```python
from build123d import *

# Parameters (mm, degrees)
SCHIZZO1_R          = 7
ESTRUSIONE1_DEPTH   = 20
SCHIZZO2_R          = 6
ESTRUSIONE2_DEPTH   = 12
ESTRUSIONE3_DEPTH   = 8
SCHIZZO4_OUTSIDE_W  = 31.456
SCHIZZO4_OUTSIDE_H  = 33.832
SCHIZZO4_OUTSIDE_R  = 5.5
ESTRUSIONE4_DEPTH   = 4
SMUSSO1_SIZE        = 0.5
SMUSSO1_EDGE_2_SIZE = 0.5
SMUSSO1_EDGE_3_SIZE = 0.5
SMUSSO1_EDGE_4_SIZE = 0.5
SMUSSO1_EDGE_5_SIZE = 0.5
SMUSSO1_EDGE_6_SIZE = 0.5
SMUSSO2_SIZE        = 1
RACCORDO1_R         = 2
RACCORDO2_R         = 0.5
SMUSSO3_SIZE        = 1


with BuildPart() as part:
    # Schizzo1 → Estrusione1 (new body)
    with BuildSketch(Plane(origin=(0, 0, 0), x_dir=(0, 0, -1), z_dir=(1, 0, 0))):
        Circle(SCHIZZO1_R)
    extrude(amount=ESTRUSIONE1_DEPTH)

    # Schizzo2 → Estrusione2 (add)
    with BuildSketch(Plane(origin=(20, 0, 0), x_dir=(0, 0, -1), z_dir=(1, 0, 0))):
        Circle(SCHIZZO2_R)
    extrude(amount=ESTRUSIONE2_DEPTH)

    # Schizzo3 → Estrusione3 (add)
    with BuildSketch(Plane.ZY):
        Polygon((9.208732283, -5.960921327), (9.766675441, 4.99453543), (0.557943158, 10.955456758), (-9.208732283, 5.960921327), (-9.766675441, -4.99453543), (-0.557943158, -10.955456758), align=None)
    extrude(amount=ESTRUSIONE3_DEPTH)

    # Schizzo4 outside → Estrusione4 (cut)
    with BuildSketch(Plane(origin=(0, 0, 0), x_dir=(0, 0, -1), z_dir=(1, 0, 0))):
        Rectangle(SCHIZZO4_OUTSIDE_W, SCHIZZO4_OUTSIDE_H)
        Circle(SCHIZZO4_OUTSIDE_R, mode=Mode.SUBTRACT)
    extrude(amount=ESTRUSIONE4_DEPTH, mode=Mode.SUBTRACT)

    # Smusso1
    smusso1_edges = [part.edges().sort_by_distance(p)[0] for p in [
        (-4, -5.960921327, 9.208732283),
    ]]
    chamfer(smusso1_edges, length=SMUSSO1_SIZE)

    # Smusso1 edge 2
    smusso1_edge_2_edges = [part.edges().sort_by_distance(p)[0] for p in [
        (-4, 4.99453543, 9.766675441),
    ]]
    chamfer(smusso1_edge_2_edges, length=SMUSSO1_EDGE_2_SIZE)

    # Smusso1 edge 3
    smusso1_edge_3_edges = [part.edges().sort_by_distance(p)[0] for p in [
        (-4, 10.955456758, 0.557943158),
    ]]
    chamfer(smusso1_edge_3_edges, length=SMUSSO1_EDGE_3_SIZE)

    # Smusso1 edge 4
    smusso1_edge_4_edges = [part.edges().sort_by_distance(p)[0] for p in [
        (-4, 5.960921327, -9.208732283),
    ]]
    chamfer(smusso1_edge_4_edges, length=SMUSSO1_EDGE_4_SIZE)

    # Smusso1 edge 5
    smusso1_edge_5_edges = [part.edges().sort_by_distance(p)[0] for p in [
        (-4, -4.99453543, -9.766675441),
    ]]
    chamfer(smusso1_edge_5_edges, length=SMUSSO1_EDGE_5_SIZE)

    # Smusso1 edge 6
    smusso1_edge_6_edges = [part.edges().sort_by_distance(p)[0] for p in [
        (-4, -10.955456758, -0.557943158),
    ]]
    chamfer(smusso1_edge_6_edges, length=SMUSSO1_EDGE_6_SIZE)

    # Smusso2
    smusso2_edges = [part.edges().sort_by_distance(p)[0] for p in [
        (0, -8.458189042, 4.325394563),
        (-8, -8.458189042, 4.325394563),
        (0, -7.974996094, -5.162309299),
        (0, 0.483192949, -9.487703862),
        (0, 8.458189042, -4.325394563),
        (0, 7.974996094, 5.162309299),
        (0, -0.483192949, 9.487703862),
        (0, 4.880709257, 9.544091519),
        (0, -5.825071083, 8.998863965),
        (0, 10.70578034, 0.545227554),
        (0, 5.825071083, -8.998863965),
        (0, -4.880709257, -9.544091519),
        (0, -10.70578034, -0.545227554),
        (-8, -7.974996094, -5.162309299),
        (-8, -0.483192949, 9.487703862),
        (-8, 7.974996094, 5.162309299),
        (-8, 8.458189042, -4.325394563),
        (-8, 0.483192949, -9.487703862),
        (-8, 4.880709257, 9.544091519),
        (-8, -5.825071083, 8.998863965),
        (-8, 10.70578034, 0.545227554),
        (-8, 5.825071083, -8.998863965),
        (-8, -4.880709257, -9.544091519),
        (-8, -10.70578034, -0.545227554),
    ]]
    chamfer(smusso2_edges, length=SMUSSO2_SIZE)

    # Raccordo1
    raccordo1_edges = [part.edges().sort_by_distance(p)[0] for p in [
        (0, 0, 5.5),
    ]]
    fillet(raccordo1_edges, radius=RACCORDO1_R)

    # Raccordo2
    raccordo2_edges = [part.edges().sort_by_distance(p)[0] for p in [
        (4, 0, 5.5),
        (20, 0, 6),
    ]]
    fillet(raccordo2_edges, radius=RACCORDO2_R)

    # Smusso3
    smusso3_edges = [part.edges().sort_by_distance(p)[0] for p in [
        (32, 0, 6),
    ]]
    chamfer(smusso3_edges, length=SMUSSO3_SIZE)


solid = part.part
```
Part model, mm, in its own coordinate system. A direction names the side the tool comes from. Coordinates: 2 decimals unless noted, no trailing zeros. Write each loop counter-clockwise with the first axis right and the second up, starting at its lowest first coordinate (ties: lowest second). Pieces come first, ordered by that corner, then holes.
Item 1: Slice it at A-A (x = -4.5). Write the cut outline in (y, z), and give its area (3 significant figures).
Item 2: Slice it at C-C (x = 13.5). Write the cut outline in (y, z), and give its area (3 significant figures).
Item 3: Pin check, flat tips, straight feed: pin 1 (5 mm diameter, centred on y = 3, z = -7.5, fed in from +X); pin 2 (2 mm diameter, centred on y = -3.5, z = -6, fed in from +X); pin 3 (2 mm diameter, centred on x = 4, z = -2.5, fed in from +Y). Stop position of each tip, or through.
Item 4: Probe line 1 (X direction, y = -5, z = 8); line 2 (Z direction, x = 19, y = 5.5); line 3 (Y direction, x = 20.5, z = 2.5). List the from-to ranges inside material, lowest first.
Item 5: Mould opens along X. For faces 1 (the face through (4, 2, -6)), 2 (the face through (-7.4, -5.6, 8.67)), 3 (the face through (-3.96, -8.49, 4.26)), 4 (the face through (-0.618, -5.612, 8.682)) say: released by +X, released by -X, zero draft, split by the parting line, or undercut.
Item 6: Which spindle directions (+Z, -Z, +X, -X, +Y, -Y) get a long thin tool onto all of the face, cutting with end or side? Do faces 5 (the face through (0, 7, 4)), 6 (the face through (-3.958, -10.706, -0.539)). Say none if no direction does.
Item 7: Slice it at B-B (y = 0). Write the cut outline in (x, z).
Results found:
1. outline: (-10.73, -0.11) - (-10.68, -0.98) - (-5.27, -9.35) - (-4.5, -9.74) - (5.46, -9.23) - (6.19, -8.76) - (10.73, 0.11) - (10.68, 0.98) - (5.27, 9.35) - (4.5, 9.74) - (-5.46, 9.23) - (-6.19, 8.76) - close
1. area: 312 mm2
2. outline: circle Ø14 at (0, 0)
2. area: 154 mm2
3. pin 1: stops at x = 31.42
3. pin 2: stops at x = 31.05
3. pin 3: stops at y = 6.84
4. line 1: x = -8 to 0
4. line 2: z = -4.33 to 4.33
4. line 3: y = -5.45 to 5.45
5. face 1: undercut
5. face 2: released by -X
5. face 3: zero draft
5. face 4: released by +X
6. face 5: +X
6. face 6: -Z, +X, -X, -Y
7. outline: (-8, -8.51) - (-7, -9.51) - (-1, -9.51) - (0, -8.51) - (0, -7.5) arc R2 cw to (2, -5.5) - (3.5, -5.5) arc R0.5 cw to (4, -6) - (4, -7) - (20, -7) - (20, -6.5) arc R0.5 cw to (20.5, -6) - (31, -6) - (32, -5) - (32, 5) - (31, 6) - (20.5, 6) arc R0.5 cw to (20, 6.5) - (20, 7) - (4, 7) - (4, 6) arc R0.5 cw to (3.5, 5.5) - (2, 5.5) arc R2 cw to (0, 7.5) - (0, 8.51) - (-1, 9.51) - (-7, 9.51) - (-8, 8.51) - close
